For this review, take the finished solid that the model builds, in its own axes (mm). Give positions to 0.01 mm unless a question says otherwise; leave off trailing zeros. Order: outer loops, then holes, each group sorted by start corner. A loop starts at its lowest first (then second) coordinate and runs counter-clockwise, first axis right, second up.
from build123d import *

# Parameters (mm, degrees)
SKETCH1_W           = 81.8
SKETCH1_H           = 102
BOSS_EXTRUDE1_DEPTH = 1.5
SKETCH2_W           = 10.6
SKETCH2_H           = 3
SKETCH2_W_2         = 6.445
SKETCH2_R           = 1.5
CUT_EXTRUDE1_DEPTH  = 2.5
CUT_EXTRUDE2_DEPTH  = 2.5
FILLET1_R           = 5


with BuildPart() as part:
    # Sketch1 → Boss-Extrude1 (new body)
    with BuildSketch(Plane.XY):
        with Locations((40.9, 51)):
            Rectangle(SKETCH1_W, SKETCH1_H)
    extrude(amount=BOSS_EXTRUDE1_DEPTH)

    # Sketch2 → Cut-Extrude1 (cut, through all)
    with BuildSketch(Plane.XY.offset(1.5)):
        with Locations((5.3, 1.5)):
            Rectangle(SKETCH2_W, SKETCH2_H)
        with Locations((44.1225, 1.5)):
            Rectangle(SKETCH2_W_2, SKETCH2_H)
        with Locations((37.6775, 1.5)):
            Rectangle(SKETCH2_W_2, SKETCH2_H)
        with Locations((76.5, 1.5)):
            Rectangle(SKETCH2_W, SKETCH2_H)
        with Locations((6, 96)):
            Circle(SKETCH2_R)
        with Locations((75.8, 96)):
            Circle(SKETCH2_R)
    extrude(amount=-CUT_EXTRUDE1_DEPTH, mode=Mode.SUBTRACT)

    # Sketch3 → Cut-Extrude2 (cut, through all)
    with BuildSketch(Plane.XY.offset(1.5)):
        with BuildLine():
            ThreePointArc((35.4, 28.5), (39.289087297, 30.110912703), (40.9, 34))
            Line((40.9, 34), (29.9, 34))
            ThreePointArc((29.9, 34), (31.510912703, 30.110912703), (35.4, 28.5))
        make_face()
        with BuildLine():
            Line((29.9, 34), (40.9, 34))
            ThreePointArc((40.9, 34), (39.289087297, 37.889087297), (35.4, 39.5))
            ThreePointArc((35.4, 39.5), (31.510912703, 37.889087297), (29.9, 34))
        make_face()
        with BuildLine():
            ThreePointArc((46.4, 39.5), (42.510912703, 37.889087297), (40.9, 34))
            Line((40.9, 34), (51.9, 34))
            ThreePointArc((51.9, 34), (50.289087297, 37.889087297), (46.4, 39.5))
        make_face()
        with BuildLine():
            Line((51.9, 34), (40.9, 34))
            ThreePointArc((40.9, 34), (42.510912703, 30.110912703), (46.4, 28.5))
            ThreePointArc((46.4, 28.5), (50.289087297, 30.110912703), (51.9, 34))
        make_face()
        with BuildLine():
            Line((40.9, 28.5), (40.9, 34))
            ThreePointArc((40.9, 34), (39.289087297, 30.110912703), (35.4, 28.5))
            Line((35.4, 28.5), (40.9, 28.5))
        make_face()
        with BuildLine():
            ThreePointArc((46.4, 28.5), (42.510912703, 30.110912703), (40.9, 34))
            Line((40.9, 34), (40.9, 28.5))
            Line((40.9, 28.5), (46.4, 28.5))
        make_face()
        with BuildLine():
            Line((40.9, 39.5), (40.9, 34))
            ThreePointArc((40.9, 34), (42.510912703, 37.889087297), (46.4, 39.5))
            Line((46.4, 39.5), (40.9, 39.5))
        make_face()
        with BuildLine():
            ThreePointArc((35.4, 39.5), (39.289087297, 37.889087297), (40.9, 34))
            Line((40.9, 34), (40.9, 39.5))
            Line((40.9, 39.5), (35.4, 39.5))
        make_face()
    extrude(amount=-CUT_EXTRUDE2_DEPTH, mode=Mode.SUBTRACT)

    # Fillet1
    fillet1_edges = [part.edges().sort_by_distance(p)[0] for p in [
        (0, 102, 0.75),
        (81.8, 102, 0.75),
    ]]
    fillet(fillet1_edges, radius=FILLET1_R)


solid = part.part
1) Clearance check with flat-ended pins moving along their axes: pin 1 (0.8 mm diameter, centred on x = 78, z = 1, fed in from -Y); pin 2 (0.8 mm diameter, centred on y = 1, z = 1, fed in from -X); pin 3 (8 mm diameter, centred on x = 29, y = 19.5, fed in from -Z); pin 4 (1.8 mm diameter, centred on x = 6, y = 96, fed in from +Z). State where each tip first meets the part, or that it passes through.
Answer sheet:
pin 1: stops at y = 3
pin 2: stops at x = 10.6
pin 3: stops at z = 0
pin 4: passes through
2) To check wall thickness, follow line 1 (X direction, y = 96, z = 0.65); line 2 (Y direction, x = 6, z = 0.85); line 3 (Y direction, x = 73.5, z = 1.3). State the ranges of each line that lie inside material, in increasing order.
Answer sheet:
line 1: x = 0 to 4.5, 7.5 to 74.3, 77.3 to 81.8
line 2: y = 3 to 94.5, 97.5 to 102
line 3: y = 3 to 102
3) We need section A-A on z = 1.2. Give the boundary of the cut face in (x, y) (3 decimals).
Answer sheet:
outline: (0, 3) - (10.6, 3) - (10.6, 0) - (34.455, 0) - (34.455, 3) - (47.345, 3) - (47.345, 0) - (71.2, 0) - (71.2, 3) - (81.8, 3) - (81.8, 97) arc R5 ccw to (76.8, 102) - (5, 102) arc R5 ccw to (0, 97) - close; hole circle Ø3 at (6, 96); hole (35.4, 28.5) - (46.4, 28.5) arc R5.5 ccw to (46.4, 39.5) - (35.4, 39.5) arc R5.5 ccw to start; hole circle Ø3 at (75.8, 96)
4) Draft analysis for pull direction Y (two halves, no side actions). For faces 1 (the face through (40, 52, 0)), 2 (the face through (75.605, 97.487, 0.76)), 3 (the face through (80.3, 100.57, 0.76)), state which applies: +Y half, -Y half, draft (parallel to the pull), parting line (faces both ways), or undercut.
Answer sheet:
face 1: draft
face 2: undercut
face 3: +Y half
